The drawing under review shows one solid part. Ordinate dimensions are in mm from its lowest x, y, z. Coordinates: 2 decimals unless noted, no trailing zeros. Write each loop counter-clockwise with the first axis right and the second up, starting at its lowest first coordinate (ties: lowest second). Pieces come first, ordered by that corner, then holes.
1) Mouldability with a two-part tool opening along X and no side actions: class the marked faces 1, 2, 3 and 4 as released by +X, released by -X, zero draft, split by the parting line, or undercut.
2) Add section C-C, the plane z = 10.5. State the section outline as (x, y) points.
3) Add section A-A, the plane z = 100. State the section outline as (x, y) points, then the cut area to 3 significant figures.
4) For line 1 (X direction, y = 13.75, z = 50.5); line 2 (Y direction, x = 1.95, z = 10); line 3 (Z direction, x = 10.5, y = 4.75) (1 decimal), list the stretches that pass through material, from the lowest coordinate up.
5) Add section B-B, the plane y = 12.78. State the section outline as (x, z) points.
6) Add section D-D, the plane x = 17. State the section outline as (y, z) points.
7) For P1, Ø8, axis at x = 39, z = 91, coming from the +Y side; P2, Ø3, axis at x = 52.77, z = 7.07, coming from the +Y side, all flat-tipped, find the tip position at first contact; note any pin that passes through.
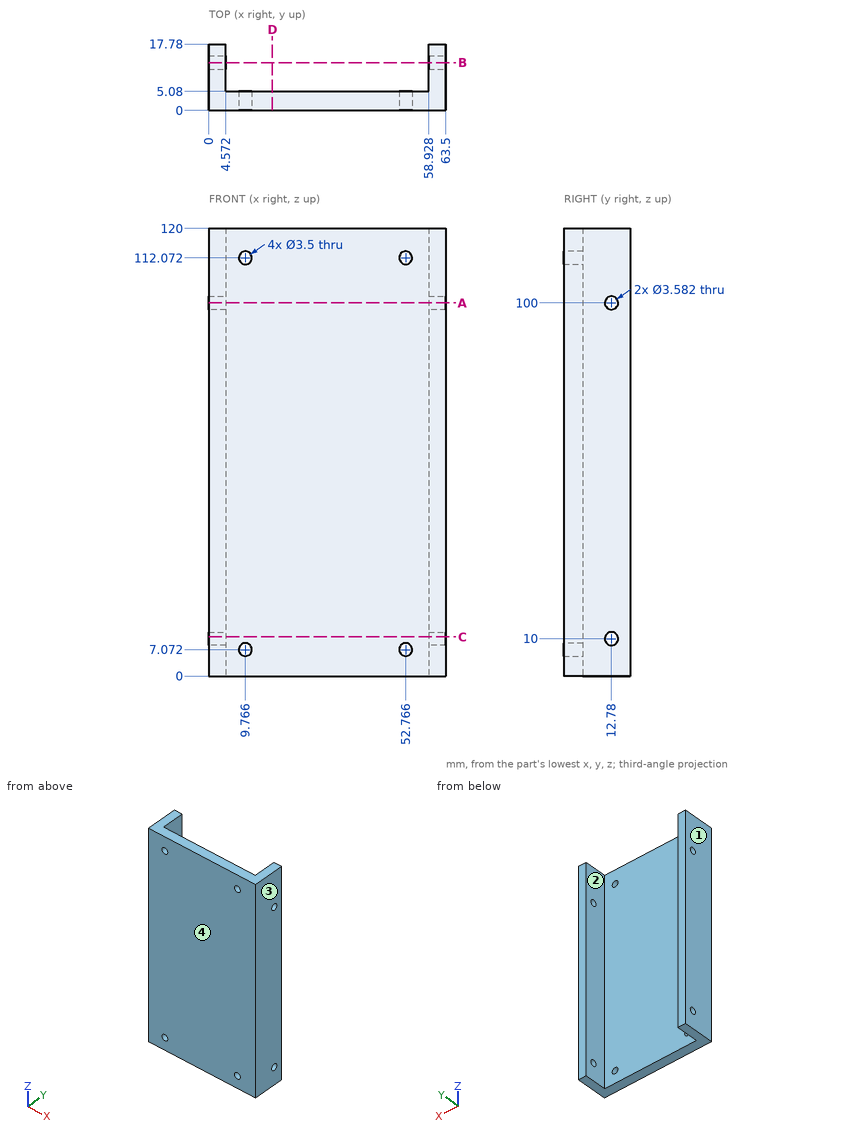
Geometry results:
1. face 1: released by -X
1. face 2: undercut
1. face 3: released by +X
1. face 4: zero draft
2. outline: (0, 0) - (63.5, 0) - (63.5, 11.06) - (58.93, 11.06) - (58.93, 5.08) - (4.57, 5.08) - (4.57, 11.06) - (0, 11.06) - close; (0, 14.5) - (4.57, 14.5) - (4.57, 17.78) - (0, 17.78) - close; (58.93, 14.5) - (63.5, 14.5) - (63.5, 17.78) - (58.93, 17.78) - close
3. outline: (0, 0) - (63.5, 0) - (63.5, 10.99) - (58.93, 10.99) - (58.93, 5.08) - (4.57, 5.08) - (4.57, 10.99) - (0, 10.99) - close; (0, 14.57) - (4.57, 14.57) - (4.57, 17.78) - (0, 17.78) - close; (58.93, 14.57) - (63.5, 14.57) - (63.5, 17.78) - (58.93, 17.78) - close
3. area: 406 mm2
4. line 1: x = 0 to 4.57, 58.93 to 63.5
4. line 2: y = 0 to 10.99, 14.57 to 17.78
4. line 3: z = 0 to 5.5, 8.7 to 110.5, 113.7 to 120
5. outline: (0, 0) - (4.57, 0) - (4.57, 8.21) - (0, 8.21) - close; (0, 11.79) - (4.57, 11.79) - (4.57, 98.21) - (0, 98.21) - close; (0, 101.79) - (4.57, 101.79) - (4.57, 120) - (0, 120) - close; (58.93, 0) - (63.5, 0) - (63.5, 8.21) - (58.93, 8.21) - close; (58.93, 11.79) - (63.5, 11.79) - (63.5, 98.21) - (58.93, 98.21) - close; (58.93, 101.79) - (63.5, 101.79) - (63.5, 120) - (58.93, 120) - close
6. outline: (0, 0) - (5.08, 0) - (5.08, 120) - (0, 120) - close
7. P1: stops at y = 5.08
7. P2: passes through
